from build123d import *

# Parameters (mm, degrees)
F0_R      = 79.375
F1_DEPTH  = 3.175
F2_R      = 73.025
F3_DEPTH  = 1.5875
F4_R      = 73.025
F5_DEPTH  = 1.5875
F6_R      = 19.05
F7_DEPTH  = 1.5875
F8_R      = 19.05
F9_DEPTH  = 25.4
F10_R     = 12.7
F11_DEPTH = 1.5875


with BuildPart() as f1:
    # F0 (on Front) → F1 (new body, symmetric)
    with BuildSketch(Plane.XZ):
        Circle(F0_R)
    extrude(amount=F1_DEPTH, both=True)

    # F2 (on face) → F3 (cut)
    with BuildSketch(Plane.XZ.offset(3.175)):
        Circle(F2_R)
    extrude(amount=-F3_DEPTH, mode=Mode.SUBTRACT)

    # F4 (on face) → F5 (cut)
    with BuildSketch(Plane(origin=(0, 3.175, 0), x_dir=(-1, 0, 0), z_dir=(0, 1, 0))):
        Circle(F4_R)
    extrude(amount=-F5_DEPTH, mode=Mode.SUBTRACT)

    # F6 (on face) → F7 (join)
    with BuildSketch(Plane.XZ.offset(1.5875)):
        Circle(F6_R)
    extrude(amount=F7_DEPTH)

    # F8 (on face) → F9 (cut)
    with BuildSketch(Plane.XZ.offset(1.5875)):
        with Locations((-23.8125, -41.24446)):
            Circle(F8_R)
        with Locations((-47.625, 0)):
            Circle(F8_R)
        with Locations((-23.8125, 41.24446)):
            Circle(F8_R)
        with Locations((23.8125, 41.24446)):
            Circle(F8_R)
        with Locations((47.625, 0)):
            Circle(F8_R)
        with Locations((23.8125, -41.24446)):
            Circle(F8_R)
    extrude(amount=-F9_DEPTH, mode=Mode.SUBTRACT)

    # F10 (on face) → F11 (join)
    with BuildSketch(Plane(origin=(0, 1.5875, 0), x_dir=(-1, 0, 0), z_dir=(0, 1, 0))):
        Circle(F10_R)
    extrude(amount=F11_DEPTH)


solid = f1.part
Geometry check sheet. Reference: the model listing, model coordinates, mm. A direction names the side the tool comes from. Give positions to 0.01 mm unless a question says otherwise; leave off trailing zeros. Write each loop counter-clockwise with the first axis right and the second up, starting at its lowest first coordinate (ties: lowest second). Pieces come first, ordered by that corner, then holes.
1) Thickness scan on line 1 (Z direction, x = 0, y = 2) (3 decimals); line 2 (Z direction, x = 0, y = -2.8) (3 decimals); line 3 (X direction, y = -0.25, z = -4). Record the ranges inside material, lowest first.
Values follow:
line 1: z = -79.375 to -73.025, -12.7 to 12.7, 73.025 to 79.375
line 2: z = -79.375 to -73.025, -19.05 to 19.05, 73.025 to 79.375
line 3: x = -79.27 to -66.25, -29 to 29, 66.25 to 79.27
2) Cross-section at D-D (z = 69). Record the boundary of the cut face in (x, y) (1 decimal).
Values follow:
outline: (-39.2, -3.2) - (-23.9, -3.2) - (-23.9, -1.6) - (23.9, -1.6) - (23.9, -3.2) - (39.2, -3.2) - (39.2, 3.2) - (23.9, 3.2) - (23.9, 1.6) - (-23.9, 1.6) - (-23.9, 3.2) - (-39.2, 3.2) - close
3) Cross-section at A-A (z = 0). Count the separate pieces of the cut face and the enclosed holes in it, plus the area to 3 significant figures.
Values follow:
separate pieces: 3
enclosed holes: 0
area: 403 mm2
4) Set-up check for faces 1 (the face through (2.75, 2.37, -12.4)), 2 (the face through (69.653, -2.392, 21.935)), 3 (the face through (23, 3.175, -70)): record each of +Z, -Z, +X, -X, +Y, -Y from which the full face is reachable in a straight line by a thin tool's end or side.
Values follow:
face 1: +Y
face 2: -Y
face 3: +Z, -Z, +X, -X, +Y
5) Go/stop test with flat-tipped pins: pin 1 Ø3 at (y, z) = (2, -8) entering from -X; pin 2 Ø2 at (x, y) = (62, -1) entering from +Z; pin 3 Ø1.5 at (x, y) = (1, -2) entering from -Z. Record where each tip stops, or that it passes through.
Values follow:
pin 1: stops at x = -79.11
pin 2: stops at z = 50.79
pin 3: stops at z = -79.37
6) Release check for a two-part mould opening along Z. For faces 4 (the face through (0, -3.175, 0)), 5 (the face through (75.71, -0.04, 23.84)), 6 (the face through (-6.2, 0, -48.5)) record: released by +Z, released by -Z, zero draft, split by the parting line, or undercut.
Values follow:
face 4: zero draft
face 5: split by the parting line
face 6: undercut
